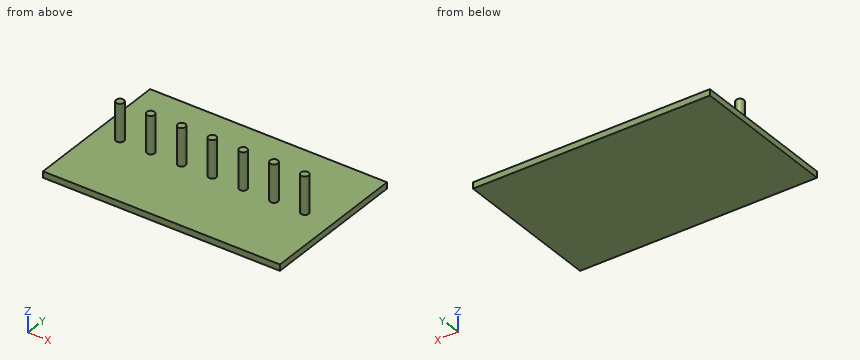
Autodesk Inventor part; units mm, degrees
ref_plane "YZ Plane" through (0, 0, 0) normal (1, 0, 0) x (0, 1, 0)
ref_plane "XZ Plane" through (0, 0, 0) normal (0, 1, 0) x (-1, 0, 0)
ref_plane "XY Plane" through (0, 0, 0) normal (0, 0, 1) x (1, 0, 0)
sketch "Sketch1" plane through (0, 0, 0) normal (0, 0, 1) x (1, 0, 0)
  line L0 (-22.1112, 10.3171) -> (130.2888, 10.3171)
  line L1 (130.2888, 10.3171) -> (130.2888, -65.8829)
  line L2 (130.2888, -65.8829) -> (-22.1112, -65.8829)
  line L3 (-22.1112, -65.8829) -> (-22.1112, 10.3171)
  point P0 (0, 0)
  dimension "d0" = 152.4
  dimension "d1" = 76.2
extrude "Extrusion1" add sketch "Sketch1" along normal blind 3.175
sketch "Sketch2" plane through (0, 0, 3.175) normal (0, 0, 1) x (1, 0, 0)
  circle A0 centre (-10.0607, -27.9271) radius 2
  circle A1 centre (5.6233, -27.9271) radius 2
  circle A2 centre (21.3073, -27.9271) radius 2
  circle A3 centre (36.9913, -27.9271) radius 2
  circle A4 centre (52.6753, -27.9271) radius 2
  circle A5 centre (68.3593, -27.9271) radius 2
  circle A6 centre (84.0433, -27.9271) radius 2
  point P0 (0, 0)
  dimension "d4" = 4
  dimension "d5" = 4
  dimension "d6" = 4
  dimension "d7" = 11.684
  dimension "d8" = 11.684
  dimension "d9" = 4
  dimension "d10" = 11.684
  dimension "d11" = 4
  dimension "d12" = 4
  dimension "d13" = 4
  dimension "d14" = 11.684
  dimension "d15" = 11.684
  dimension "d16" = 11.684
extrude "Extrusion2" add sketch "Sketch2" along normal blind 19.05
sketch "Sketch3" plane through (130.2888, -65.8829, 0) normal (1, 0, 0) x (0, 0, -1)
  line L0 (-11.1509, 83.1688) -> (7.2167, 83.1688)
  line L1 (7.2167, 83.1688) -> (7.2167, -5.5026)
  line L2 (7.2167, -5.5026) -> (-11.1509, -5.5026)
  line L3 (-11.1509, -5.5026) -> (-11.1509, 83.1688)
  point P0 (0, 65.8829)
extrude "Extrusion3" cut sketch "Sketch3" against normal blind 31.75
properties part number "gearbasephonecase"
Geometry: final body of the model. Coordinates: model frame, mm. Round coordinates to 2 decimals unless told otherwise and drop trailing zeros. Order: outer loops, then holes, each group sorted by start corner. A loop starts at its lowest first (then second) coordinate and runs counter-clockwise, first axis right, second up. Notation, with made-up numbers: (82, -15.75) -> (141, -15.75) arc R31 ccw to (141, 11.25) -> close; hole circle Ø9 at (-29, 52.25). An arc over 180 degrees is marked (long way). Use one line per item in the form item = value.
(1) Ray query, probe 1 along Z at (x, y) = (51, -40.5) (3 decimals); probe 2 along Y at (x, z) = (5, 14.75). Return the intervals inside material, ascending. Write a range as [from, to].
Results list:
probe_1 = [0, 3.175]
probe_2 = [-29.83, -26.03]
(2) First-contact query: pin 1 Ø12 at (x, y) = (43.5, -2.5) entering from +Z (3 decimals); pin 2 Ø2 at (x, z) = (38.5, 18) entering from -Y; pin 3 Ø3 at (x, z) = (52.5, 13.5) entering from +Y. Flat tips, straight axial feed; report the tip coordinate or a pass-through.
Results list:
pin_1 = 3.175
pin_2 = -29.86
pin_3 = -25.93
(3) Section C-C on x = 0.5. Return loops of the section in (y, z) (3 decimals).
Results list:
outline = (-65.883, 0) -> (10.317, 0) -> (10.317, 3.175) -> (-65.883, 3.175) -> close
(4) Section A-A on z = 9.75. Return loops of the section in (x, y), and give its area (3 significant figures).
Results list:
outline = circle Ø4 at (-10.06, -27.93); circle Ø4 at (5.62, -27.93); circle Ø4 at (21.31, -27.93); circle Ø4 at (36.99, -27.93); circle Ø4 at (52.68, -27.93); circle Ø4 at (68.36, -27.93); circle Ø4 at (84.04, -27.93)
area = 88.0 mm^2
(5) Section B-B on y = -17. Return loops of the section in (x, z) (3 decimals), and give its area (3 significant figures).
Results list:
outline = (-22.111, 0) -> (98.539, 0) -> (98.539, 3.175) -> (-22.111, 3.175) -> close
area = 383 mm^2
